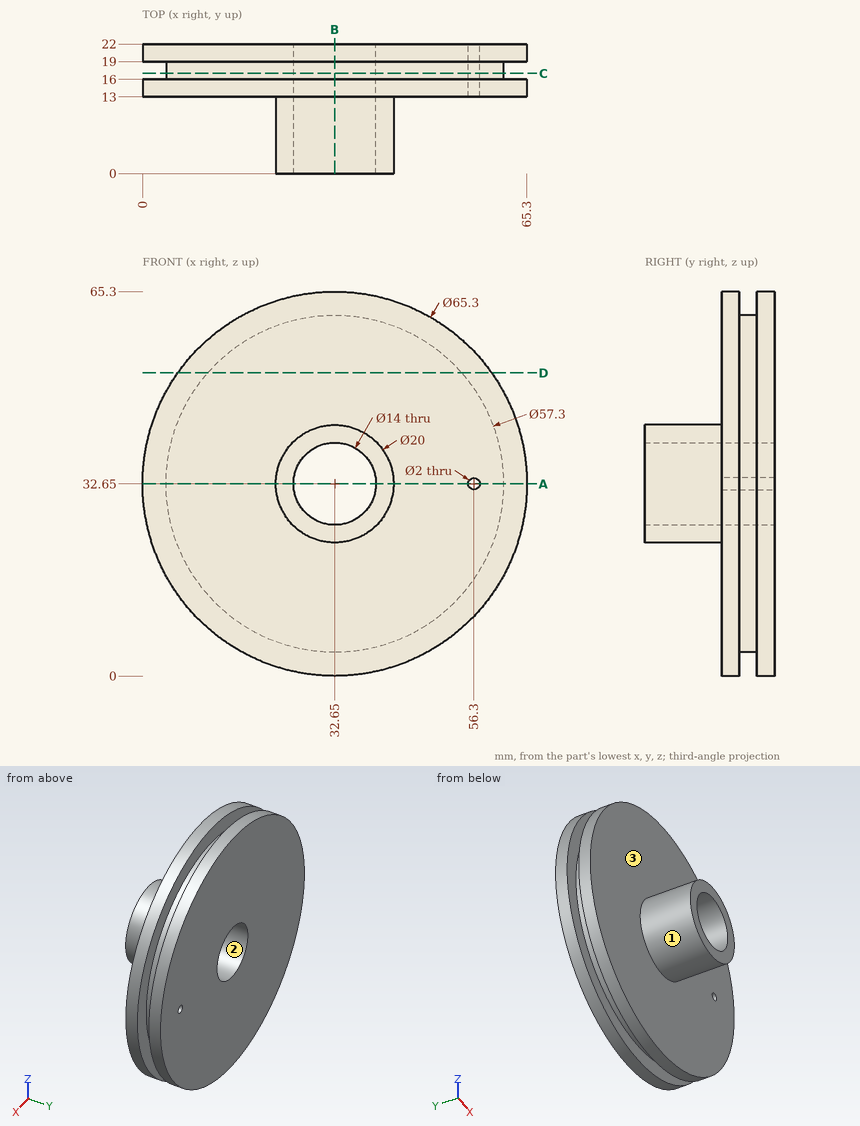
Source: three-view drawing plus pictorial views. Frame: mm from the lowest corner of the part. Round coordinates to 2 decimals unless told otherwise and drop trailing zeros. Loops run counter-clockwise (first coordinate to the right, second up) from the corner with the lowest first, then second, coordinate; pieces in that order, holes last. Notation, with made-up numbers: (79.5, 68.25) - (111.5, 68.25) arc R19 ccw to (111.5, 81.25) - close; hole circle Ø3 at (67.5, 22.5). An arc over 180 degrees is marked (long way). Write item = value, one per line. Start each with the question number.
Item 1: Material intervals for line 1 (X direction, y = 16.25, z = 32.65); line 2 (X direction, y = 20.25, z = 32.65); line 3 (Z direction, x = 32.65, y = 9.75), sorted ascending.
Item 2: Mould query, pull axis Z, two halves, no side actions, for the marked faces 1, 2 and 3. Classes: released by +Z, released by -Z, zero draft, split by the parting line, or undercut.
Item 3: Section query B-B on x = 32.65. Output: boundary loops of the cut face in (y, z).
Item 4: Section query D-D on z = 51.5. Output: boundary loops of the cut face in (x, y).
Item 5: Section query A-A on z = 32.65. Output: boundary loops of the cut face in (x, y), plus the area to 3 significant figures.
Item 6: Section query C-C on y = 17. Output: boundary loops of the cut face in (x, z).
Item 7: First-contact query: pin 1 Ø10 at (x, y) = (51, 13.5) entering from +Z; pin 2 Ø3 at (y, z) = (15.5, 24.5) entering from -X; pin 3 Ø2 at (x, y) = (45.5, 3) entering from +Z; pin 4 Ø10 at (x, y) = (38.5, 8.5) entering from +Z. Flat tips, straight axial feed; report the tip coordinate or a pass-through.
Results list:
q1.line_1 = 4 to 25.65, 39.65 to 55.3, 57.3 to 61.3
q1.line_2 = 0 to 25.65, 39.65 to 55.3, 57.3 to 65.3
q1.line_3 = 22.65 to 25.65, 39.65 to 42.65
q2.face_1 = split by the parting line
q2.face_2 = undercut
q2.face_3 = zero draft
q3.outline = (0, 22.65) - (13, 22.65) - (13, 0) - (16, 0) - (16, 4) - (19, 4) - (19, 0) - (22, 0) - (22, 25.65) - (0, 25.65) - close; (0, 39.65) - (22, 39.65) - (22, 65.3) - (19, 65.3) - (19, 61.3) - (16, 61.3) - (16, 65.3) - (13, 65.3) - (13, 42.65) - (0, 42.65) - close
q4.outline = (5.99, 13) - (59.31, 13) - (59.31, 16) - (54.23, 16) - (54.23, 19) - (59.31, 19) - (59.31, 22) - (5.99, 22) - (5.99, 19) - (11.07, 19) - (11.07, 16) - (5.99, 16) - close
q5.outline = (0, 13) - (22.65, 13) - (22.65, 0) - (25.65, 0) - (25.65, 22) - (0, 22) - (0, 19) - (4, 19) - (4, 16) - (0, 16) - close; (39.65, 0) - (42.65, 0) - (42.65, 13) - (55.3, 13) - (55.3, 22) - (39.65, 22) - close; (57.3, 13) - (65.3, 13) - (65.3, 16) - (61.3, 16) - (61.3, 19) - (65.3, 19) - (65.3, 22) - (57.3, 22) - close
q5.area = 498 mm²
q6.outline = circle Ø57.3 at (32.65, 32.65); hole circle Ø14 at (32.65, 32.65); hole circle Ø2 at (56.3, 32.65)
q7.pin_1 = 62.45
q7.pin_2 = 0.68
q7.pin_3 = through
q7.pin_4 = 65.09
